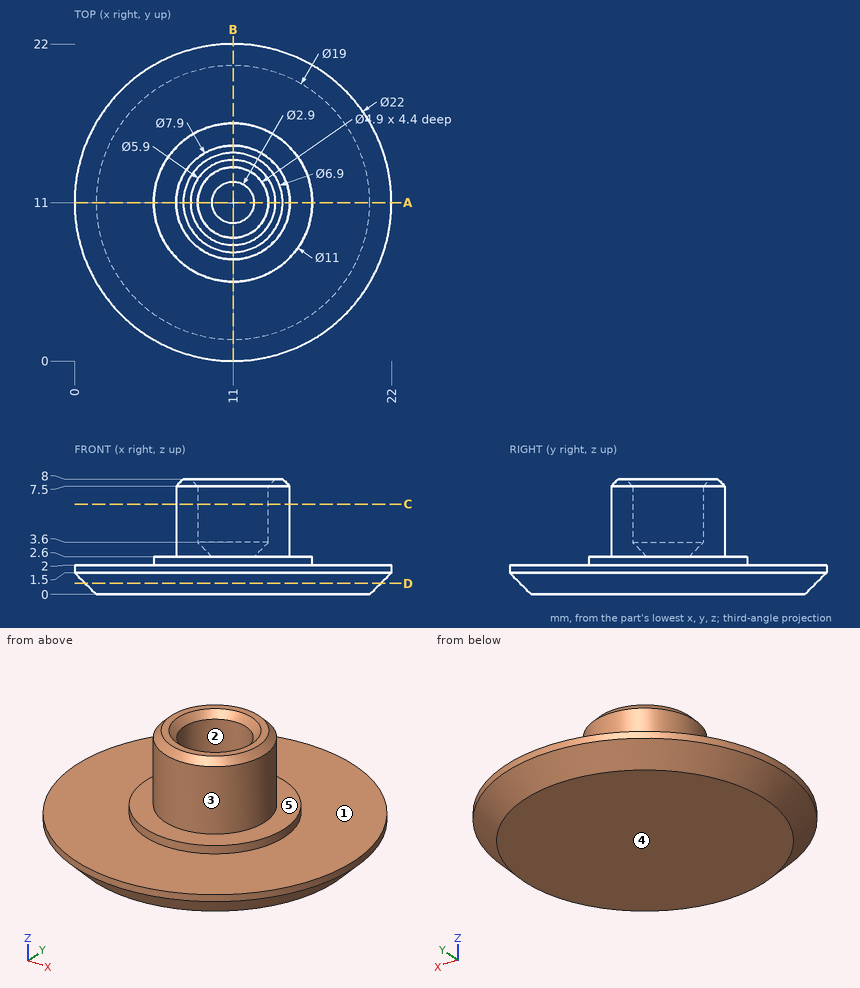
Here's the drawing with two shaded views (mm, measured from the low corner). I have some questions. A direction names the side the tool comes from. Give positions to 0.01 mm unless a question says otherwise; leave off trailing zeros. Order: outer loops, then holes, each group sorted by start corner. A loop starts at its lowest first (then second) coordinate and runs counter-clockwise, first axis right, second up. Notation, with made-up numbers: (0, -9) -> (45, -9) arc R9 ccw to (45, 4) -> close; hole circle Ø8 at (10.25, 50.25). An arc over 180 degrees is marked (long way). One line per item, written item: value. Start each with the question number.
1. Will these pins go through, and if not, where does the flat tip stop? pin 1 Ø10 at (x, y) = (11.5, 15.5) entering from +Z; pin 2 Ø6.5 at (x, y) = (5.5, 15) entering from +Z; pin 3 Ø1.5 at (y, z) = (19, 4.5) entering from -X; pin 4 Ø3 at (x, y) = (11, 11) entering from +Z.
2. We'd pull the mould along X, two halves only. Please class the marked faces 1, 2 and 3: released by +X, released by -X, zero draft, split by the parting line, or undercut.
3. I need wall thicknesses on probe 1 along Y at (x, z) = (11, 4.95); probe 2 along Z at (x, y) = (18.25, 6.5). Which ranges of each line are inside material? Lowest first, please. Write a range as from..to.
4. Imagine slicing it at D-D, the plane z = 0.75. List the corners of the cut face in (x, y) for me.
5. For the marked faces 4 and 5, which set-ups out of +Z, -Z, +X, -X, +Y, -Y let a thin tool reach every point of the face, with its end or its side?
6. Imagine slicing it at C-C, the plane z = 6.25. List the corners of the cut face in (x, y) for me, plus the area to 3 significant figures.
7. Imagine slicing it at A-A, the plane y = 11. List the corners of the cut face in (x, z) for me, plus the area to 4 significant figures.
Values follow:
1. pin 1: stops at z = 8
1. pin 2: stops at z = 7.9
1. pin 3: passes through
1. pin 4: stops at z = 2.65
2. face 1: zero draft
2. face 2: undercut
2. face 3: split by the parting line
3. probe 1: y = 7.05..8.55, 13.45..14.95
3. probe 2: z = 0..2
4. outline: circle Ø20.5 at (11, 11)
5. face 4: -Z, +X, -X, +Y, -Y
5. face 5: +Z
6. outline: circle Ø7.9 at (11, 11); hole circle Ø4.9 at (11, 11)
6. area: 30.2 mm2
7. outline: (0, 1.5) -> (1.5, 0) -> (20.5, 0) -> (22, 1.5) -> (22, 2) -> (16.5, 2) -> (16.5, 2.6) -> (14.95, 2.6) -> (14.95, 7.5) -> (14.45, 8) -> (13.95, 8) -> (13.45, 7.5) -> (13.45, 3.6) -> (12.45, 2.6) -> (9.55, 2.6) -> (8.55, 3.6) -> (8.55, 7.5) -> (8.05, 8) -> (7.55, 8) -> (7.05, 7.5) -> (7.05, 2.6) -> (5.5, 2.6) -> (5.5, 2) -> (0, 2) -> close
7. area: 65.05 mm2
